```python
from build123d import *

# Parameters (mm, degrees)
F1_DEPTH       = 38.1
F3_D           = 3.7973
F3_CSINK_D     = 7.7978
F3_CSINK_ANGLE = 82
F4_R           = 5.08
F6_D           = 3.7973
F6_CSINK_D     = 7.7978
F6_CSINK_ANGLE = 82


# Not quite as in the source:
# - a pattern or mirror of a feature is missing from the dataset's text; its kind, count and spacing are read off the source's solid


with BuildPart() as f1:
    # F0 (on Right) → F1 (new body, symmetric)
    with BuildSketch(Plane.YZ):
        Polygon((30.48, 7.62), (-7.62, 7.62), (-7.62, -30.48), (0, -30.48), (0, 0), (30.48, 0), align=None)
    extrude(amount=F1_DEPTH, both=True)

    # F3 (through all)
    with Locations(Plane.XY.offset(7.62)):
        with Locations((-28.405956924, 21.6088658199), (-7.0089674555, 21.6088658199), (-17.7074621897, 6.9944329099)):
            f3 = CounterSinkHole(F3_D / 2, F3_CSINK_D / 2, counter_sink_angle=F3_CSINK_ANGLE)

    # F3_copies: F3 across plane
    add(f3.mirror(Plane(origin=(0, 0, 0), x_dir=(0, 0, 1), z_dir=(1, 0, 0))), mode=Mode.SUBTRACT)

    # F4
    f4_edges = [f1.edges().sort_by_distance(p)[0] for p in [
        (0, -7.62, 7.62),
    ]]
    fillet(f4_edges, radius=F4_R)

    # F6 (through all)
    with Locations(Plane.XZ.offset(7.62)):
        with Locations((-8.0344257876, -19.893276193), (-29.0398038924, -19.893276193)):
            f6 = CounterSinkHole(F6_D / 2, F6_CSINK_D / 2, counter_sink_angle=F6_CSINK_ANGLE)

    # F6_copies: F6 across plane
    add(f6.mirror(Plane(origin=(0, 0, 0), x_dir=(0, 0, 1), z_dir=(1, 0, 0))), mode=Mode.SUBTRACT)


solid = f1.part
```
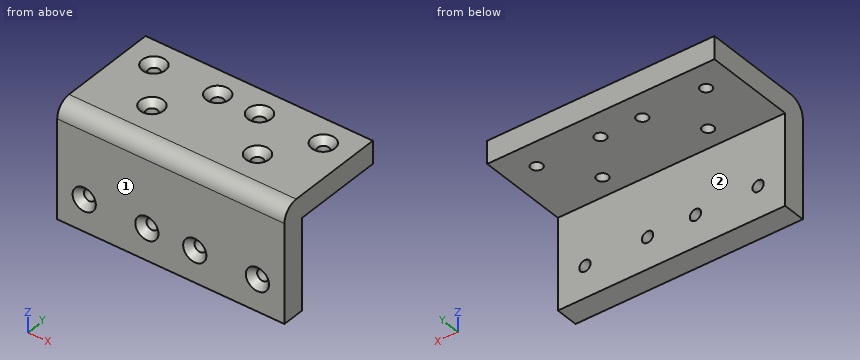
Work out the finished part from the listing and answer in its coordinate system (mm). Face numbers are marked on the shaded views. A direction names the side the tool comes from. Give positions to 0.01 mm unless a question says otherwise; leave off trailing zeros. Loops run counter-clockwise (first coordinate to the right, second up) from the corner with the lowest first, then second, coordinate; pieces in that order, holes last. Notation, with made-up numbers: (-15.5, 43.25) - (-6.5, 43.25) arc R16 cw to (-6.5, 70.25) - close; hole circle Ø11 at (66, 87.5). An arc over 180 degrees is marked (long way). Use CSV: the item, a comma, the result in double quotes. Start each with the question number.
(1) Find section B-B, the plane x = -23. Determine the outline of the cut face in (y, z).
(2) Find the intervals of material crossed by L1, parallel to X at y = 20, z = 6.5; L2, parallel to X at y = 22, z = 2; L3, parallel to Z at x = -16, y = 14, in increasing order.
(3) A tool of negligible diameter and unlimited length cuts with its end or side. For the marked faces 1 and 2, from which of +Z, -Z, +X, -X, +Y, -Y can it reach the whole face along a straight path? Write none if from no direction.
(4) Find section D-D, the plane y = 27. Determine the outline of the cut face in (x, z).
(5) Find section C-C, the plane z = -5. Determine the outline of the cut face in (x, y).
(6) Each of these flat-tipped pins is pushed along its axis until it touches: pin 1 (4.5 mm diameter, centred on x = 8.03, z = -19.89, fed in from +Y); pin 2 (5 mm diameter, centred on x = -29.04, z = -19.89, fed in from -Y); pin 3 (4.5 mm diameter, centred on x = -17.71, y = 6.99, fed in from -Z). Where does it stop, or does it pass through?
(7) Find section A-A, the plane z = 4. Determine the outline of the cut face in (x, y), plus the area to 3 significant figures.
Results found:
1,outline,"(-7.62, -30.48) - (0, -30.48) - (0, 0) - (30.48, 0) - (30.48, 7.62) - (-2.54, 7.62) arc R5.08 ccw to (-7.62, 2.54) - close"
2,L1,"-38.1 to -30.85, -25.96 to -9.45, -4.57 to 4.57, 9.45 to 25.96, 30.85 to 38.1"
2,L2,"-38.1 to -30.26, -26.55 to -8.87, -5.15 to 5.15, 8.87 to 26.55, 30.26 to 38.1"
2,L3,"0 to 7.62"
3,face 1,"+Z, -Z, +X, -X, -Y"
3,face 2,"-Z, +X, -X, +Y"
4,outline,"(-38.1, 0) - (38.1, 0) - (38.1, 7.62) - (-38.1, 7.62) - close"
5,outline,"(-38.1, -7.62) - (38.1, -7.62) - (38.1, 0) - (-38.1, 0) - close"
6,pin 1,"y = 0"
6,pin 2,"y = -6.01"
6,pin 3,"z = 0"
7,outline,"(-38.1, -7.41) - (38.1, -7.41) - (38.1, 30.48) - (-38.1, 30.48) - close; hole circle Ø3.8 at (-28.41, 21.61); hole circle Ø3.8 at (-17.71, 6.99); hole circle Ø3.8 at (-7.01, 21.61); hole circle Ø3.8 at (7.01, 21.61); hole circle Ø3.8 at (17.71, 6.99); hole circle Ø3.8 at (28.41, 21.61)"
7,area,"2,820 mm^2"
